Autodesk Inventor part; units mm, degrees
ref_plane "YZ Plane" through (0, 0, 0) normal (1, 0, 0) x (0, 1, 0)
ref_plane "XZ Plane" through (0, 0, 0) normal (0, 1, 0) x (-1, 0, 0)
ref_plane "XY Plane" through (0, 0, 0) normal (0, 0, 1) x (1, 0, 0)
sketch "MASTER SKETCH" plane through (0, 0, 0) normal (0, 0, 1) x (1, 0, 0)
  circle A0 centre (0, 0) radius 22.86
  circle A1 centre (-31.6504, 3.081) radius 8.89
  circle A2 centre (-31.6504, 3.081) radius 20.32
  circle A3 centre (-60.6627, 6.8802) radius 8.89
  circle A4 centre (-58.2971, 5.0584) radius 6.35
  circle A5 centre (-60.6627, 6.8802) radius 25.4
  circle A6 centre (-58.2971, 5.0584) radius 25.4 construction
  line L0 (-44.0087, 26.0584) -> (-77.3167, -12.298) construction
  line L1 (-68.9445, 30.8921) -> (-52.3809, -17.1317) construction
  circle A7 centre (-44.0087, 26.0584) radius 2
  arc A8 (-68.9445, 30.8921) -> (-69.3394, 27.9326) centre (-44.0087, 26.0584) ccw construction
  arc A9 (-70.9079, 31.2727) -> (-71.334, 28.0802) centre (-44.0087, 26.0584) ccw
  arc A10 (-66.981, 30.5115) -> (-67.3449, 27.785) centre (-44.0087, 26.0584) ccw
  arc A11 (-66.981, 30.5115) -> (-70.9079, 31.2727) centre (-68.9445, 30.8921) ccw
  arc A12 (-71.334, 28.0802) -> (-67.3449, 27.785) centre (-69.3394, 27.9326) ccw
  arc A13 (-85.5985, 11.7139) -> (-83.6279, 6.9326) centre (-44.0087, 26.0584) ccw construction
  arc A14 (-87.4892, 11.0618) -> (-85.429, 6.0631) centre (-44.0087, 26.0584) ccw
  arc A15 (-83.7078, 12.366) -> (-81.8268, 7.8021) centre (-44.0087, 26.0584) ccw
  arc A16 (-83.7078, 12.366) -> (-87.4892, 11.0618) centre (-85.5985, 11.7139) ccw
  arc A17 (-85.429, 6.0631) -> (-81.8268, 7.8021) centre (-83.6279, 6.9326) ccw
  arc A18 (-77.3167, -12.298) -> (-72.5856, -15.9416) centre (-44.0087, 26.0584) ccw construction
  arc A19 (-78.6281, -13.8081) -> (-73.7107, -17.5951) centre (-44.0087, 26.0584) ccw
  arc A20 (-76.0054, -10.7879) -> (-71.4605, -14.288) centre (-44.0087, 26.0584) ccw
  arc A21 (-76.0054, -10.7879) -> (-78.6281, -13.8081) centre (-77.3167, -12.298) ccw
  arc A22 (-73.7107, -17.5951) -> (-71.4605, -14.288) centre (-72.5856, -15.9416) ccw
  arc A23 (-52.3809, -17.1317) -> (-47.2548, -17.8157) centre (-44.0087, 26.0584) ccw construction
  arc A24 (-52.7615, -19.0951) -> (-47.4024, -19.8103) centre (-44.0087, 26.0584) ccw
  arc A25 (-52.0003, -15.1682) -> (-47.1072, -15.8212) centre (-44.0087, 26.0584) ccw
  arc A26 (-52.0003, -15.1682) -> (-52.7615, -19.0951) centre (-52.3809, -17.1317) ccw
  arc A27 (-47.4024, -19.8103) -> (-47.1072, -15.8212) centre (-47.2548, -17.8157) ccw
  arc A28 (-35.7269, 2.0465) -> (-32.9664, 3.1843) centre (-44.0087, 26.0584) ccw construction
  arc A29 (-35.0748, 0.1558) -> (-32.0969, 1.3831) centre (-44.0087, 26.0584) ccw
  arc A30 (-36.379, 3.9372) -> (-33.8358, 4.9854) centre (-44.0087, 26.0584) ccw
  arc A31 (-36.379, 3.9372) -> (-35.0748, 0.1558) centre (-35.7269, 2.0465) ccw
  arc A32 (-32.0969, 1.3831) -> (-33.8358, 4.9854) centre (-32.9664, 3.1843) ccw
  line L2 (-91.0627, 30.0584) -> (30.5868, 30.0584)
  line L3 (30.5868, 30.0584) -> (30.5868, -19.9416)
  line L4 (30.5868, -19.9416) -> (-91.0627, -19.9416)
  line L5 (-91.0627, -19.9416) -> (-91.0627, 30.0584)
  circle A33 centre (0, 0) radius 14.2875 construction
  circle A34 centre (25.5868, -14.9416) radius 3
  circle A35 centre (25.5868, 25.0584) radius 3
  circle A36 centre (-51.8755, -14.9416) radius 3
  line L6 (-91.0627, 25.3566) -> (30.5868, 25.3566) construction
  circle A37 centre (-15.8118, 25.0584) radius 3
  line L7 (-58.2971, 5.0584) -> (-60.6627, 6.8802) construction
  line L8 (-52.3328, 12.803) -> (-54.6984, 14.6248)
  line L9 (-66.627, -0.8643) -> (-64.2614, -2.6861)
  arc A38 (-64.2614, -2.6861) -> (-52.3328, 12.803) centre (-58.2971, 5.0584) ccw
  arc A39 (-54.6984, 14.6248) -> (-66.627, -0.8643) centre (-60.6627, 6.8802) ccw
  circle A40 centre (0, 0) radius 24.13 construction
  circle A41 centre (-31.6504, 3.081) radius 21.59 construction
  line L10 (-67.5422, -2.0527) -> (-65.1767, -3.8745)
  arc A42 (-65.1767, -3.8745) -> (-51.4176, 13.9914) centre (-58.2971, 5.0584) ccw
  line L11 (-51.4176, 13.9914) -> (-53.7832, 15.8132)
  arc A43 (-53.7832, 15.8132) -> (-67.5422, -2.0527) centre (-60.6627, 6.8802) ccw
  circle A44 centre (-44.0087, 26.0584) radius 50.8 construction
  arc A45 (-67.3815, -0.857) -> (-64.0616, -3.4137) centre (-44.0087, 26.0584) ccw
  arc A46 (-53.9439, 14.6174) -> (-52.5326, 13.5306) centre (-44.0087, 26.0584) ccw
  arc A47 (-53.9439, 14.6174) -> (-67.3815, -0.857) centre (-60.6627, 6.8802) ccw
  arc A48 (-64.0616, -3.4137) -> (-52.5326, 13.5306) centre (-58.2971, 5.0584) ccw
  line L12 (-35.7269, 2.0465) -> (-85.5985, 11.7139) construction
  point P0 (-60.0285, -7.7006)
  point P1 (-59.4799, 5.9693)
  dimension "d0" = 45.72
  dimension "d1" = 17.78
  dimension "d2" = 40.64
  dimension "d4" = 17.78
  dimension "d5" = 12.7
  dimension "d6" = 50.8
  dimension "d9" = 50.8
  dimension "d10" = 60
  dimension "d12" = 4
  dimension "d13" = 4
  dimension "d14" = 4
  dimension "d15" = 4
  dimension "d16" = 4
  dimension "d17" = 4
  dimension "d19" = 28.575
  dimension "d28" = 6
  dimension "d29" = 6
  dimension "d30" = 6
  dimension "d39" = 31.8
  dimension "d42" = 29.26
  dimension "d43" = 26.72
  dimension "d70" = 2
  dimension "d73" = 6
  dimension "d84" = 2
  dimension "d85" = 5
  dimension "d89" = 19.55
  dimension "d108" = 1.27
  dimension "d109" = 1.27
  dimension "d110" = 2.5
  dimension "d111" = 2.5
  dimension "d113" = 2.5
  dimension "d114" = 2
  dimension "d129" = 1.5
  dimension "d133" = 2.5
  dimension "d136" = 50
  dimension "d139" = 2
  dimension "d140" = 2.5
  dimension "d141" = 2
  dimension "d142" = 2
  dimension "d181" = 60
sketch "Sketch2" plane through (0, 0, 0) normal (0, 0, 1) x (1, 0, 0)
  line L0 (-91.0627, 30.0584) -> (30.5868, 30.0584)
  line L1 (-91.0627, -19.9416) -> (-91.0627, 30.0584)
  line L2 (30.5868, 30.0584) -> (30.5868, -19.9416)
  line L3 (30.5868, -19.9416) -> (-91.0627, -19.9416)
  line L4 (-91.0627, 30.0584) -> (30.5868, 30.0584)
  line L5 (30.5868, 30.0584) -> (30.5868, -19.9416)
  line L6 (30.5868, -19.9416) -> (-91.0627, -19.9416)
  line L7 (-91.0627, -19.9416) -> (-91.0627, 30.0584)
  point P0 (0, 0)
extrude "Extrusion1" add sketch "Sketch2" along normal blind 5
sketch "Sketch3" plane through (0, 0, 0) normal (0, 0, -1) x (-1, 0, 0)
  arc A0 (47.1072, -15.8212) -> (47.4024, -19.8103) centre (47.2548, -17.8157) ccw
  arc A1 (47.1072, -15.8212) -> (52.0003, -15.1682) centre (44.0087, 26.0584) ccw
  arc A2 (47.4024, -19.8103) -> (52.7615, -19.0951) centre (44.0087, 26.0584) ccw
  arc A3 (52.7615, -19.0951) -> (52.0003, -15.1682) centre (52.3809, -17.1317) ccw
  line L0 (91.0627, 30.0584) -> (91.0627, -19.9416)
  line L1 (-30.5868, 30.0584) -> (91.0627, 30.0584)
  line L2 (-30.5868, -19.9416) -> (-30.5868, 30.0584)
  line L3 (91.0627, -19.9416) -> (-30.5868, -19.9416)
  arc A4 (71.4605, -14.288) -> (73.7107, -17.5951) centre (72.5856, -15.9416) ccw
  arc A5 (73.7107, -17.5951) -> (78.6281, -13.8081) centre (44.0087, 26.0584) ccw
  arc A6 (71.4605, -14.288) -> (76.0054, -10.7879) centre (44.0087, 26.0584) ccw
  arc A7 (78.6281, -13.8081) -> (76.0054, -10.7879) centre (77.3167, -12.298) ccw
  arc A8 (81.8268, 7.8021) -> (83.7078, 12.366) centre (44.0087, 26.0584) ccw
  arc A9 (81.8268, 7.8021) -> (85.429, 6.0631) centre (83.6279, 6.9326) ccw
  arc A10 (85.429, 6.0631) -> (87.4892, 11.0618) centre (44.0087, 26.0584) ccw
  arc A11 (87.4892, 11.0618) -> (83.7078, 12.366) centre (85.5985, 11.7139) ccw
  arc A12 (71.334, 28.0802) -> (70.9079, 31.2727) centre (44.0087, 26.0584) ccw
  arc A13 (67.3449, 27.785) -> (66.981, 30.5115) centre (44.0087, 26.0584) ccw
  arc A14 (70.9079, 31.2727) -> (66.981, 30.5115) centre (68.9445, 30.8921) ccw
  arc A15 (67.3449, 27.785) -> (71.334, 28.0802) centre (69.3394, 27.9326) ccw
  arc A16 (66.627, -0.8643) -> (54.6984, 14.6248) centre (60.6627, 6.8802) ccw
  arc A17 (52.3328, 12.803) -> (64.2614, -2.6861) centre (58.2971, 5.0584) ccw
  line L4 (52.3328, 12.803) -> (54.6984, 14.6248)
  line L5 (66.627, -0.8643) -> (64.2614, -2.6861)
  point P0 (0, 0)
extrude "Extrusion2" cut sketch "Sketch3" against normal blind 5 contours A6 A7 A5 A4 | A8 A11 A10 A9 | L5 A17 L4 A16
sketch "Sketch4" plane through (0, 0, 0) normal (0, 0, -1) x (-1, 0, 0)
  circle A0 centre (-25.5868, 25.0584) radius 3
  circle A1 centre (15.8118, 25.0584) radius 3
  circle A2 centre (51.8755, -14.9416) radius 3
  circle A3 centre (-25.5868, -14.9416) radius 3
  point P0 (0, 0)
sketch "Sketch5" plane through (0, 0, 0) normal (0, 0, -1) x (-1, 0, 0)
  circle A0 centre (0, 0) radius 22.86
hole "Hole1" at (0, 0, 0) direction (0, 0, 1) diameter 28.575 end through all
hole "Hole2" at (25.5868, 25.0584, 0) at (-15.8118, 25.0584, 0) at (25.5868, -14.9416, 0) at (-51.8755, -14.9416, 0) direction (0, 0, 1) diameter 4.5 end through all counterbore diameter 6 counterbore depth 1
sketch "Sketch6" plane through (0, 0, 0) normal (0, 0, -1) x (-1, 0, 0)
  line L0 (91.0627, 25.3566) -> (-30.5868, 25.3566) construction
  circle A0 centre (44.0087, 26.0584) radius 2
  point P0 (0, 0)
hole "Hole3" at (-44.0087, 26.0584, 0) direction (0, 0, 1) diameter 4 end through all
sketch "Sketch7" plane through (0, 0, 0) normal (0, 0, -1) x (-1, 0, 0)
  circle A0 centre (31.6504, 3.081) radius 20.32
  point P0 (0, 0)
hole "Hole4" at (-31.6504, 3.081, 0) direction (0, 0, 1) diameter 8 depth 5 counterbore diameter 22 counterbore depth 3
sketch "Sketch8" plane through (0, 0, 0) normal (0, 0, -1) x (-1, 0, 0)
  arc A0 (52.3328, 12.803) -> (64.2614, -2.6861) centre (58.2971, 5.0584) ccw
  line L0 (66.627, -0.8643) -> (64.2614, -2.6861)
  arc A1 (66.627, -0.8643) -> (54.6984, 14.6248) centre (60.6627, 6.8802) ccw
  line L1 (52.3328, 12.803) -> (54.6984, 14.6248)
  arc A2 (67.5422, -2.0527) -> (53.7832, 15.8132) centre (60.6627, 6.8802) ccw
  line L2 (51.4176, 13.9914) -> (53.7832, 15.8132)
  line L3 (67.5422, -2.0527) -> (65.1767, -3.8745)
  arc A3 (51.4176, 13.9914) -> (65.1767, -3.8745) centre (58.2971, 5.0584) ccw
  point P0 (0, 0)
extrude "Extrusion3" cut sketch "Sketch8" against normal blind 1 contours L1 A1 L0 A0 | L3 A3 L2 A2
sketch "Sketch11" plane through (0, 0, 0) normal (0, 0, 1) x (1, 0, 0)
  line L0 (30.5868, -19.9416) -> (30.5868, 30.0584)
  line L1 (30.5868, 30.0584) -> (30.5868, -19.9416)
  line L2 (30.5868, -19.9416) -> (-61.3292, -19.9416)
  line L3 (-91.0627, -19.9416) -> (30.5868, -19.9416)
  line L4 (-61.3292, -19.9416) -> (-32.4617, 30.0584)
  line L5 (30.5868, 30.0584) -> (-91.0627, 30.0584)
  line L6 (-32.4617, 30.0584) -> (30.5868, 30.0584)
  circle A0 centre (-44.0087, 26.0584) radius 2
  point P0 (0, 0)
  dimension "d147" = 120
  dimension "d148" = 8
extrude "Extrusion5" [suppressed]
sketch "Sketch12" plane through (0, 0, 0) normal (0, 0, 1) x (1, 0, 0)
  circle A0 centre (-15.8118, 25.0584) radius 3
  circle A1 centre (25.5868, 25.0584) radius 3
  circle A2 centre (25.5868, -14.9416) radius 3
  circle A3 centre (-51.8755, -14.9416) radius 3
  point P0 (0, 0)
hole "Hole5" [suppressed]
sketch "Sketch13" plane through (0, 0, 0) normal (0, 0, 1) x (1, 0, 0)
  circle A0 centre (0, 0) radius 14.2875 construction
hole "Hole6" [suppressed]
sketch "Sketch14" plane through (0, 0, 0) normal (0, 0, 1) x (1, 0, 0)
  circle A0 centre (-31.6504, 3.081) radius 8.89
  point P0 (0, 0)
hole "Hole7" [suppressed]
sketch "Sketch15" plane through (0, 0, 5) normal (0, 0, 1) x (1, 0, 0)
  circle A0 centre (-15.8118, 25.0584) radius 2.25
  circle A1 centre (-51.8755, -14.9416) radius 2.25
  circle A2 centre (25.5868, 25.0584) radius 2.25
  circle A3 centre (25.5868, -14.9416) radius 2.25
  point P0 (0, 0)
hole "Hole8" at (-15.8118, 25.0584, 5) at (-51.8755, -14.9416, 5) at (25.5868, -14.9416, 5) at (25.5868, 25.0584, 5) direction (0, 0, -1) diameter 4 end through all countersink diameter 8 countersink angle 90
sketch "Sketch16" plane through (0, 0, 0) normal (0, 0, -1) x (-1, 0, 0)
  circle A0 centre (44.0087, 26.0584) radius 2
  arc A1 (67.5422, -2.0527) -> (53.7832, 15.8132) centre (60.6627, 6.8802) ccw
  line L0 (51.4176, 13.9914) -> (53.7832, 15.8132)
  arc A2 (51.4176, 13.9914) -> (65.1767, -3.8745) centre (58.2971, 5.0584) ccw
  line L1 (67.5422, -2.0527) -> (65.1767, -3.8745)
  arc A3 (71.4605, -14.288) -> (76.0054, -10.7879) centre (44.0087, 26.0584) ccw
  arc A4 (78.6281, -13.8081) -> (76.0054, -10.7879) centre (77.3167, -12.298) ccw
  arc A5 (73.7107, -17.5951) -> (78.6281, -13.8081) centre (44.0087, 26.0584) ccw
  arc A6 (71.4605, -14.288) -> (73.7107, -17.5951) centre (72.5856, -15.9416) ccw
  line L2 (58.1824, 5.2073) -> (44.0087, 26.0584)
  point P0 (0, 0)
  dimension "d180" = 2.9858
equation "\"d0\" = SR2PD"
equation "\"d1\" = SR1PD"
equation "\"d2\" = FirstReductionPD"
equation "\"d4\" = Pinion4inPD"
equation "\"d5\" = PinionPD"
equation "\"PinionPD\" = 12.7"
equation "\"FirstReductionPD\" = 40.64"
equation "\"HighGearPD\" = 20.32"
equation "\"LowGearPD\" = 17.78"
equation "\"HighGearDogPD\" = 63.5"
equation "\"LowGearDogPD\" = 76.2"
equation "\"SR1PD\" = 17.78"
equation "\"SR2PD\" = 45.72"
equation "\"Pinion4inPD\" = 17.78"
properties part number "GEARBOX BACKPLATE" material "Aluminum 6061"
The listing builds one solid part. Answer for the finished solid, in the listing's coordinates (mm). A direction names the side the tool comes from. Round coordinates to 2 decimals unless told otherwise and drop trailing zeros. Write each loop counter-clockwise with the first axis right and the second up, starting at its lowest first coordinate (ties: lowest second). Pieces come first, ordered by that corner, then holes. Notation, with made-up numbers: M 79,-24.5 L 96,-24.5 A22 ccw 96,9.5 Z; hole C 23,-22.5 d10. An arc over 180 degrees is marked long. Write each question's results on one line, items separated by ' | '. Start each with the question number.
Item 1: Find section B-B on x = -29. Write down the section's boundary in (y, z).
Item 2: Find section A-A on x = 0. Write down the section's boundary in (y, z), and give its area (3 significant figures).
Item 3: The mould has two halves that part along Y. Classify faces 4 (the cylindrical face through (-82.72, 5.15, 2.46)), 5 (the flat face through (-91.063, 5, 2)), 6 (the cylindrical face through (-17.71, 26.27, 2.14)): +Y half, -Y half, draft (parallel to the pull), parting line (faces both ways), or undercut.
Item 4: Given pin 1 Ø11 at (x, y) = (-28.5, 7.5) entering from -Z; pin 2 Ø5 at (x, y) = (-15.81, 25.06) entering from +Z; pin 3 Ø6 at (x, y) = (-51.88, -14.94) entering from +Z, each flat-ended and moving along its own axis, determine where each tip first touches the part or whether it passes through.
Item 5: Straight lines are drawn through the part: probe 1 along X at (y, z) = (0, 3.6); probe 2 along X at (y, z) = (2.5, 1.8); probe 3 along X at (y, z) = (7.5, 0.85). For each, find the intervals that lie inside material, in ascending order.
Item 6: Which of the six approach directions +Z, -Z, +X, -X, +Y, -Y give full straight-line access (tool end or side, diameter ignored) to faces 1 (the flat face through (-18, 24, 1)), 2 (the flat face through (-65.461, -1.762, 2.972)), 3 (the flat face through (-31, 17, 0))?
Answer block:
1) outline: M -19.94,0 L -7.59,0 L -7.59,3 L 0.09,3 L 0.09,5 L -19.94,5 Z; M 6.08,3 L 13.76,3 L 13.76,0 L 30.06,0 L 30.06,5 L 6.08,5 Z
2) outline: M -19.94,0 L -14.29,0 L -14.29,5 L -19.94,5 Z; M 14.29,0 L 30.06,0 L 30.06,5 L 14.29,5 Z | area: 107 mm²
3) face 4: undercut | face 5: draft | face 6: undercut
4) pin 1: stops at z = 3 | pin 2: stops at z = 3.5 | pin 3: stops at z = 4
5) probe 1: x = -91.06 to -67.61, -49.93 to -34.2, -29.1 to -14.29, 14.29 to 30.59 | probe 2: x = -91.06 to -69.4, -48.86 to -42.64, -20.67 to -14.07, 14.07 to 30.59 | probe 3: x = -91.06 to -86.09, -81.71 to -71.92, -47.29 to -41.72, -21.58 to -12.16, 12.16 to 30.59
6) face 1: -Z | face 2: +Z, -Z | face 3: -Z, +X, -X, +Y, -Y
